```python
from build123d import *

# Parameters (mm, degrees)
F0_R     = 185
F1_DEPTH = 20
F4_R     = 2.5
F5_DEPTH = 5


# Not quite as in the source:
# - the program builds the solid bodies; features that only make, move or delete a surface that nothing else refers to are left out


with BuildPart() as f1:
    # F0 (on Top) → F1 (new body)
    with BuildSketch(Plane.XY):
        Circle(F0_R)
    extrude(amount=F1_DEPTH)

    # F4 (on face) → F5 (cut)
    with BuildSketch(Plane.XY.offset(20)):
        Circle(F4_R)
        with Locations((0, 25)):
            Circle(F4_R)
        with Locations((0, 50)):
            Circle(F4_R)
        with Locations((0, 75)):
            Circle(F4_R)
        with Locations((0, 100)):
            Circle(F4_R)
        with Locations((0, 125)):
            Circle(F4_R)
        with Locations((25, 0)):
            Circle(F4_R)
        with Locations((25, 25)):
            Circle(F4_R)
        with Locations((25, 50)):
            Circle(F4_R)
        with Locations((25, 75)):
            Circle(F4_R)
        with Locations((25, 100)):
            Circle(F4_R)
        with Locations((25, 125)):
            Circle(F4_R)
        with Locations((50, 0)):
            Circle(F4_R)
        with Locations((50, 25)):
            Circle(F4_R)
        with Locations((50, 50)):
            Circle(F4_R)
        with Locations((50, 75)):
            Circle(F4_R)
        with Locations((50, 100)):
            Circle(F4_R)
        with Locations((50, 125)):
            Circle(F4_R)
        with Locations((75, 0)):
            Circle(F4_R)
        with Locations((75, 25)):
            Circle(F4_R)
        with Locations((75, 50)):
            Circle(F4_R)
        with Locations((75, 75)):
            Circle(F4_R)
        with Locations((75, 100)):
            Circle(F4_R)
        with Locations((75, 125)):
            Circle(F4_R)
        with Locations((100, 0)):
            Circle(F4_R)
        with Locations((100, 25)):
            Circle(F4_R)
        with Locations((100, 50)):
            Circle(F4_R)
        with Locations((100, 75)):
            Circle(F4_R)
        with Locations((100, 100)):
            Circle(F4_R)
        with Locations((125, 0)):
            Circle(F4_R)
        with Locations((125, 25)):
            Circle(F4_R)
        with Locations((125, 50)):
            Circle(F4_R)
        with Locations((125, 75)):
            Circle(F4_R)
        with Locations((75, -25)):
            Circle(F4_R)
        with Locations((100, -50)):
            Circle(F4_R)
        with Locations((0, -100)):
            Circle(F4_R)
        with Locations((100, -100)):
            Circle(F4_R)
        with Locations((75, -100)):
            Circle(F4_R)
        with Locations((125, -50)):
            Circle(F4_R)
        with Locations((75, -125)):
            Circle(F4_R)
        with Locations((25, -50)):
            Circle(F4_R)
        with Locations((0, -75)):
            Circle(F4_R)
        with Locations((100, -75)):
            Circle(F4_R)
        with Locations((100, -25)):
            Circle(F4_R)
        with Locations((50, -125)):
            Circle(F4_R)
        with Locations((125, -25)):
            Circle(F4_R)
        with Locations((50, -75)):
            Circle(F4_R)
        with Locations((25, -25)):
            Circle(F4_R)
        with Locations((75, -75)):
            Circle(F4_R)
        with Locations((75, -50)):
            Circle(F4_R)
        with Locations((125, -75)):
            Circle(F4_R)
        with Locations((0, -125)):
            Circle(F4_R)
        with Locations((25, -75)):
            Circle(F4_R)
        with Locations((50, -100)):
            Circle(F4_R)
        with Locations((25, -125)):
            Circle(F4_R)
        with Locations((0, -50)):
            Circle(F4_R)
        with Locations((25, -100)):
            Circle(F4_R)
        with Locations((50, -25)):
            Circle(F4_R)
        with Locations((50, -50)):
            Circle(F4_R)
        with Locations((0, -25)):
            Circle(F4_R)
        with Locations((-25, -75)):
            Circle(F4_R)
        with Locations((-50, -100)):
            Circle(F4_R)
        with Locations((-100, 0)):
            Circle(F4_R)
        with Locations((-100, -100)):
            Circle(F4_R)
        with Locations((-100, -75)):
            Circle(F4_R)
        with Locations((-50, -125)):
            Circle(F4_R)
        with Locations((-125, -75)):
            Circle(F4_R)
        with Locations((-50, -25)):
            Circle(F4_R)
        with Locations((-75, 0)):
            Circle(F4_R)
        with Locations((-75, -100)):
            Circle(F4_R)
        with Locations((-25, -100)):
            Circle(F4_R)
        with Locations((-125, -50)):
            Circle(F4_R)
        with Locations((-25, -125)):
            Circle(F4_R)
        with Locations((-75, -50)):
            Circle(F4_R)
        with Locations((-25, -25)):
            Circle(F4_R)
        with Locations((-75, -75)):
            Circle(F4_R)
        with Locations((-50, -75)):
            Circle(F4_R)
        with Locations((-75, -125)):
            Circle(F4_R)
        with Locations((-125, 0)):
            Circle(F4_R)
        with Locations((-75, -25)):
            Circle(F4_R)
        with Locations((-100, -50)):
            Circle(F4_R)
        with Locations((-125, -25)):
            Circle(F4_R)
        with Locations((-50, 0)):
            Circle(F4_R)
        with Locations((-100, -25)):
            Circle(F4_R)
        with Locations((-25, -50)):
            Circle(F4_R)
        with Locations((-50, -50)):
            Circle(F4_R)
        with Locations((-25, 0)):
            Circle(F4_R)
        with Locations((-75, 25)):
            Circle(F4_R)
        with Locations((-100, 50)):
            Circle(F4_R)
        with Locations((-100, 100)):
            Circle(F4_R)
        with Locations((-75, 100)):
            Circle(F4_R)
        with Locations((-125, 50)):
            Circle(F4_R)
        with Locations((-75, 125)):
            Circle(F4_R)
        with Locations((-25, 50)):
            Circle(F4_R)
        with Locations((-100, 75)):
            Circle(F4_R)
        with Locations((-100, 25)):
            Circle(F4_R)
        with Locations((-50, 125)):
            Circle(F4_R)
        with Locations((-125, 25)):
            Circle(F4_R)
        with Locations((-50, 75)):
            Circle(F4_R)
        with Locations((-25, 25)):
            Circle(F4_R)
        with Locations((-75, 75)):
            Circle(F4_R)
        with Locations((-75, 50)):
            Circle(F4_R)
        with Locations((-125, 75)):
            Circle(F4_R)
        with Locations((-25, 75)):
            Circle(F4_R)
        with Locations((-50, 100)):
            Circle(F4_R)
        with Locations((-25, 125)):
            Circle(F4_R)
        with Locations((-25, 100)):
            Circle(F4_R)
        with Locations((-50, 25)):
            Circle(F4_R)
        with Locations((-50, 50)):
            Circle(F4_R)
    extrude(amount=-F5_DEPTH, mode=Mode.SUBTRACT)


solid = f1.part
```
Design review of the part built by this model. Coordinates are the model's own, in mm. Coordinates: 2 decimals unless noted, no trailing zeros. Write each loop counter-clockwise with the first axis right and the second up, starting at its lowest first coordinate (ties: lowest second). Pieces come first, ordered by that corner, then holes.
1) Add section A-A (y = 147). Write out the cut boundary in (x, z), plus the area to 3 significant figures.
2) Add section B-B (z = 9). Write out the cut boundary in (x, y).
3) Insertion check: pin 1 (6.5 mm diameter, centred on x = 25, y = 125, fed in from +Z); pin 2 (1 mm diameter, centred on x = 66.5, z = 16, fed in from +Y); pin 3 (1.5 mm diameter, centred on x = -4, z = 11, fed in from +Y); pin 4 (2.5 mm diameter, centred on x = 24.5, y = -0.5, fed in from +Z). Each pin has a flat end and moves straight along its axis. Give the tip position at first contact, or say it passes through.
4) Add section C-C (x = 65.5). Write out the cut boundary in (y, z), plus the area to 3 significant figures.
5) To check wall thickness, follow L1, parallel to Y at x = 8, z = 3; L2, parallel to Y at x = 72, z = 5; L3, parallel to X at y = 156, z = 10.5. State the ranges of each line that lie inside material, in increasing order.
Check result:
1. outline: (-112.32, 0) - (112.32, 0) - (112.32, 20) - (-112.32, 20) - close
1. area: 4,490 mm2
2. outline: circle Ø370 at (0, 0)
3. pin 1: stops at z = 20
3. pin 2: stops at y = 172.83
3. pin 3: stops at y = 184.97
3. pin 4: stops at z = 15
4. outline: (-173.02, 0) - (173.02, 0) - (173.02, 20) - (-173.02, 20) - close
4. area: 6,920 mm2
5. L1: y = -184.83 to 184.83
5. L2: y = -170.41 to 170.41
5. L3: x = -99.44 to 99.44
